from build123d import *

# Parameters (mm, degrees)
BOSS_EXTRUDE1_DEPTH = 76.2
SKETCH5_W           = 152.4
SKETCH5_H           = 170.103674112
BOSS_EXTRUDE3_DEPTH = 12.7
SKETCH6_W           = 152.4
SKETCH6_H           = 170.103674112
BOSS_EXTRUDE4_DEPTH = 12.7


with BuildPart() as part:
    # Sketch2 → Boss-Extrude1 (new body)
    with BuildSketch(Plane(origin=(0, 0, 0), x_dir=(0, 0, -1), z_dir=(1, 0, 0))):
        Polygon((0, 0), (0, 170.103674112), (1193.8, 762), (1193.8, 591.896325888), align=None)
    extrude(amount=BOSS_EXTRUDE1_DEPTH)

    # Sketch5 → Boss-Extrude3 (add)
    with BuildSketch(Plane(origin=(0, 0, -1193.8), x_dir=(-1, 0, 0), z_dir=(0, 0, -1))):
        with Locations((-76.2, 676.948162944)):
            Rectangle(SKETCH5_W, SKETCH5_H)
    extrude(amount=BOSS_EXTRUDE3_DEPTH)

    # Sketch6 → Boss-Extrude4 (add)
    with BuildSketch(Plane.XY):
        with Locations((76.2, 85.051837056)):
            Rectangle(SKETCH6_W, SKETCH6_H)
    extrude(amount=BOSS_EXTRUDE4_DEPTH)


solid = part.part
Model file for the job. Use its own axes, mm. A direction names the side the tool comes from. Round coordinates to 2 decimals unless told otherwise and drop trailing zeros. Loops run counter-clockwise (first coordinate to the right, second up) from the corner with the lowest first, then second, coordinate; pieces in that order, holes last.
1. Band-saw the part on B-B, the plane x = 23. List the corners of the cut face in (y, z), and give its area (3 significant figures).
Check values:
outline: (0, 0) - (591.9, -1193.8) - (591.9, -1206.5) - (762, -1206.5) - (762, -1193.8) - (170.1, 0) - (170.1, 12.7) - (0, 12.7) - close
area: 207,000 mm2
2. Band-saw the part on D-D, the plane z = -887. List the corners of the cut face in (x, y), and give its area (3 significant figures).
Check values:
outline: (0, 439.78) - (76.2, 439.78) - (76.2, 609.89) - (0, 609.89) - close
area: 13,000 mm2
3. Band-saw the part on A-A, the plane x = 121. List the corners of the cut face in (y, z), and give its area (3 significant figures).
Check values:
outline: (0, 0) - (170.1, 0) - (170.1, 12.7) - (0, 12.7) - close; (591.9, -1206.5) - (762, -1206.5) - (762, -1193.8) - (591.9, -1193.8) - close
area: 4,320 mm2
4. Wall check: probe 1 along Z at (x, y) = (124, 729.5); probe 2 along X at (y, z) = (384, -460.5); probe 3 along Z at (x, y) = (137.5, 78). Give the ranges that are in metal, low to high.
Check values:
probe 1: z = -1206.5 to -1193.8
probe 2: x = 0 to 76.2
probe 3: z = 0 to 12.7
5. Drop flat-ended pins along their axis: P1, Ø5, axis at x = 79, y = 633, coming from the +Z side; P2, Ø14, axis at x = 57, z = 8.5, coming from the +Y side; P3, Ø4, axis at x = 77.5, z = -1199.5, coming from the -Y side. Give the stop position or say it passes through.
Check values:
P1: stops at z = -1193.8
P2: stops at y = 170.1
P3: stops at y = 591.9
6. Tool access for faces 1 (the flat face through (115, 678, -1193.8)), 2 (the flat face through (114, 86, 0)), 3 (the flat face through (76.2, 383, -600)), 4 (the flat face through (0, 407, -600)): list every direction of +Z, -Z, +X, -X, +Y, -Y with a clear straight run to the whole face (end or side of a thin tool).
Check values:
face 1: +Z, +X, +Y, -Y
face 2: -Z, +X, +Y, -Y
face 3: +X, +Y, -Y
face 4: +Z, -Z, -X, +Y, -Y
7. Band-saw the part on C-C, the plane y = 662. List the corners of the cut face in (x, z), and give its area (3 significant figures).
Check values:
outline: (0, -1206.5) - (152.4, -1206.5) - (152.4, -1193.8) - (76.2, -1193.8) - (76.2, -992.11) - (0, -992.11) - close
area: 17,300 mm2
